Geometry: see drawing. Coordinates: mm, zero at the bounding-box minimum. Give positions to 0.01 mm unless a question says otherwise; leave off trailing zeros. Write each loop counter-clockwise with the first axis right and the second up, starting at its lowest first coordinate (ties: lowest second). Pieces come first, ordered by that corner, then holes. Notation, with made-up numbers: (-20, -22.5) -> (-9, -22.5) arc R11 cw to (-9, -8.5) -> close; hole circle Ø7 at (30.5, 4.25). An arc over 180 degrees is marked (long way). Write item = value, one per line.
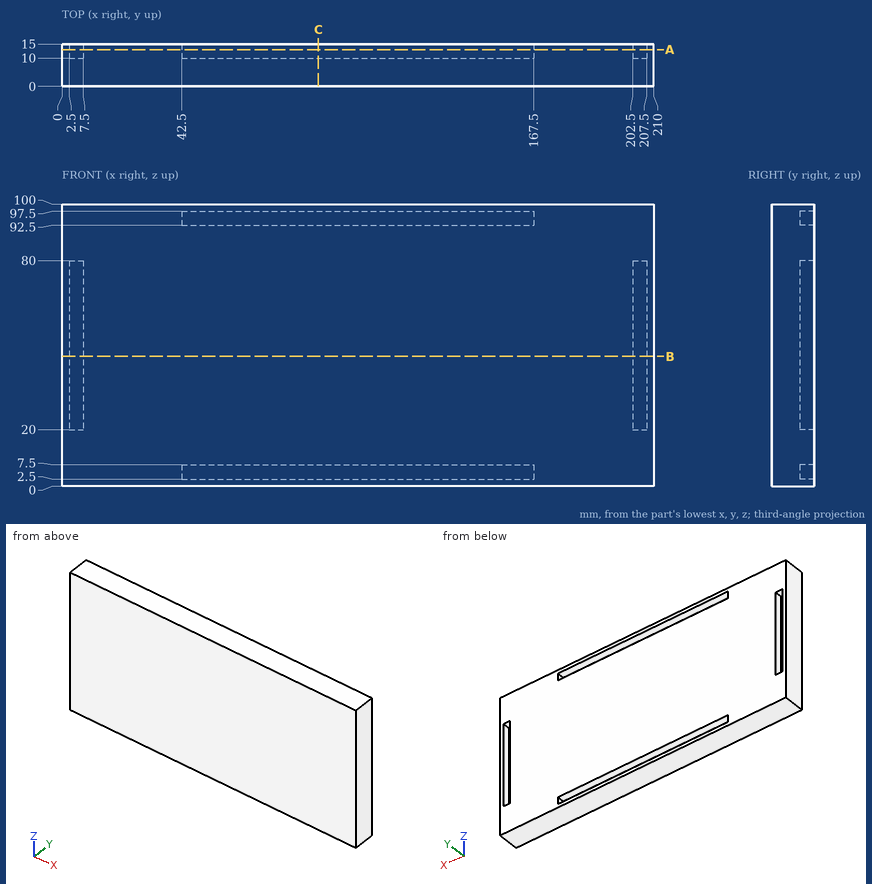
(1) First-contact query: pin 1 (1.5 mm diameter, centred on x = 6, z = 63.5, fed in from +Y). Flat tip, straight axial feed; report the tip coordinate or a pass-through.
Values follow:
pin_1 = 10
(2) Material intervals for line 1 (Z direction, x = 119.5, y = 14.5); line 2 (X direction, y = 10.5, z = 95.5), sorted ascending.
Values follow:
line_1 = 0 to 2.5, 7.5 to 92.5, 97.5 to 100
line_2 = 0 to 42.5, 167.5 to 210
(3) Section query C-C (x = 91). Return loops of the section in (y, z), plus the area to 3 significant figures.
Values follow:
outline = (0, 0) -> (15, 0) -> (15, 2.5) -> (10, 2.5) -> (10, 7.5) -> (15, 7.5) -> (15, 92.5) -> (10, 92.5) -> (10, 97.5) -> (15, 97.5) -> (15, 100) -> (0, 100) -> close
area = 1,450 mm2
(4) Section query B-B (z = 46). Return loops of the section in (x, y), plus the area to 3 significant figures.
Values follow:
outline = (0, 0) -> (210, 0) -> (210, 15) -> (207.5, 15) -> (207.5, 10) -> (202.5, 10) -> (202.5, 15) -> (7.5, 15) -> (7.5, 10) -> (2.5, 10) -> (2.5, 15) -> (0, 15) -> close
area = 3,100 mm2
(5) Section query A-A (y = 13). Return loops of the section in (x, z).
Values follow:
outline = (0, 0) -> (210, 0) -> (210, 100) -> (0, 100) -> close; hole (2.5, 20) -> (7.5, 20) -> (7.5, 80) -> (2.5, 80) -> close; hole (42.5, 2.5) -> (167.5, 2.5) -> (167.5, 7.5) -> (42.5, 7.5) -> close; hole (42.5, 92.5) -> (167.5, 92.5) -> (167.5, 97.5) -> (42.5, 97.5) -> close; hole (202.5, 20) -> (207.5, 20) -> (207.5, 80) -> (202.5, 80) -> close
